from build123d import *

# Parameters (mm, degrees)
SKETCH_1_W          = 50
SKETCH_1_H          = 27
EXTRUDE_1_DEPTH     = 35
SKETCH_2_W          = 50
SKETCH_2_H          = 21
CUT_EXTRUDE_1_DEPTH = 15
SKETCH_3_R          = 1.6
CUT_EXTRUDE_2_DEPTH = 53.758784453
SKETCH_4_W          = 14
SKETCH_4_H          = 21
CUT_EXTRUDE_3_DEPTH = 63.544986529


with BuildPart() as part:
    # 草图1 → 凸台-拉伸1 (new body)
    with BuildSketch(Plane.XY):
        with Locations((3.800856531, -0.170235546)):
            Rectangle(SKETCH_1_W, SKETCH_1_H)
    extrude(amount=EXTRUDE_1_DEPTH)

    # 草图2 → 切除-拉伸1 (cut)
    with BuildSketch(Plane.XY.offset(35)):
        with Locations((3.800856531, -0.170235546)):
            Rectangle(SKETCH_2_W, SKETCH_2_H)
    extrude(amount=-CUT_EXTRUDE_1_DEPTH, mode=Mode.SUBTRACT)

    # 草图3 → 切除-拉伸2 (cut, through all)
    with BuildSketch(Plane.XZ.offset(13.670235546)):
        with Locations(Location((-3.699143469, 30, 0), (0, 0, 270))):
            Circle(SKETCH_3_R)
        with Locations(Location((11.300856531, 30, 0), (0, 0, 270))):
            Circle(SKETCH_3_R)
    extrude(amount=-CUT_EXTRUDE_2_DEPTH, mode=Mode.SUBTRACT)

    # 草图4 → 切除-拉伸3 (cut, through all)
    with BuildSketch(Plane.ZY.offset(21.199143469)):
        with Locations((10, -0.170235546)):
            Rectangle(SKETCH_4_W, SKETCH_4_H)
    extrude(amount=-CUT_EXTRUDE_3_DEPTH, mode=Mode.SUBTRACT)


solid = part.part
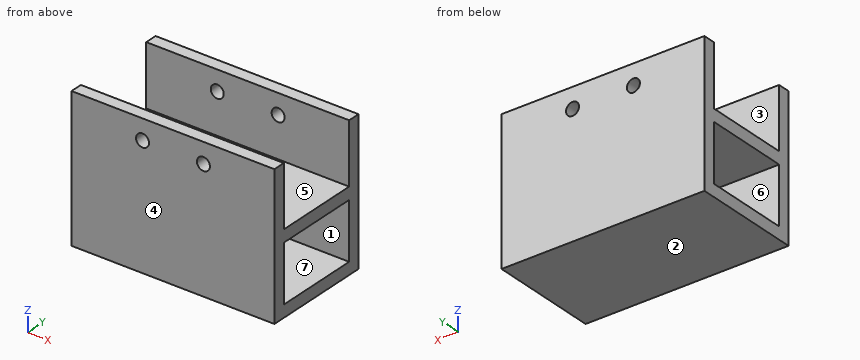
Check sheet for the modelled part. Datum: model origin and axes. Units: mm. Face numbers are marked on the shaded views. A direction names the side the tool comes from. Give positions to 0.01 mm unless a question says otherwise; leave off trailing zeros. Loops run counter-clockwise (first coordinate to the right, second up) from the corner with the lowest first, then second, coordinate; pieces in that order, holes last. Notation, with made-up numbers: M 9,10.25 L 36,10.25 A18 cw 36,43.25 Z; hole C 89.25,6.25 d2. An arc over 180 degrees is marked long. Return JSON: item names as keys, results as strings. Group by question number.
1. Thickness scan on L1, parallel to X at y = -11.5, z = 30; L2, parallel to Y at x = 2, z = 24; L3, parallel to Z at x = 18.5, y = -3. Record the ranges inside material, lowest first.
2. Cross-section at C-C on z = 30. Record the boundary of the cut face in (x, y), plus the area to 3 significant figures.
3. Mould release check, pull along Z, two halves, no side actions. Record for the marked faces 4, 5, 6 and 7: released by +Z, released by -Z, zero draft, split by the parting line, or undercut.
4. Cross-section at D-D on z = 15. Record the boundary of the cut face in (x, y).
5. Go/stop test with a flat-tipped pin: pin 1 (3 mm diameter, centred on x = -13.5, y = 8.5, fed in from +Z). Record where the tip stops, or that it passes through.
6. Cross-section at A-A on y = 5.25. Record the boundary of the cut face in (x, z).
7. Cross-section at B-B on x = 14. Record the boundary of the cut face in (y, z).
8. Tool access check on the marked faces 1, 2 and 3. Record the directions out of +Z, -Z, +X, -X, +Y, -Y that give a thin tool (end or side, any length) a straight path to the whole face; none if there is none.
Return value:
{
 "1": {"L1": "-21.2 to -5.3, -2.1 to 9.7, 12.9 to 28.8", "L2": "-13.67 to -10.67, 10.33 to 13.33", "L3": "0 to 3, 17 to 20"},
 "2": {"outline": "M -21.2,-13.67 L -5.3,-13.67 L -5.3,-10.67 L -21.2,-10.67 Z; M -21.2,10.33 L -5.3,10.33 L -5.3,13.33 L -21.2,13.33 Z; M -2.1,-13.67 L 9.7,-13.67 L 9.7,-10.67 L -2.1,-10.67 Z; M -2.1,10.33 L 9.7,10.33 L 9.7,13.33 L -2.1,13.33 Z; M 12.9,-13.67 L 28.8,-13.67 L 28.8,-10.67 L 12.9,-10.67 Z; M 12.9,10.33 L 28.8,10.33 L 28.8,13.33 L 12.9,13.33 Z", "area": "262 mm^2"},
 "3": {"face 4": "zero draft", "face 5": "released by +Z", "face 6": "undercut", "face 7": "undercut"},
 "4": {"outline": "M -21.2,-13.67 L 28.8,-13.67 L 28.8,-10.67 L -21.2,-10.67 Z; M -21.2,10.33 L 28.8,10.33 L 28.8,13.33 L -21.2,13.33 Z"},
 "5": {"pin 1": "z = 20"},
 "6": {"outline": "M -21.2,0 L 28.8,0 L 28.8,3 L -21.2,3 Z; M -21.2,17 L 28.8,17 L 28.8,20 L -21.2,20 Z"},
 "7": {"outline": "M -13.67,0 L 13.33,0 L 13.33,35 L 10.33,35 L 10.33,20 L -10.67,20 L -10.67,35 L -13.67,35 Z; hole M -10.67,3 L 10.33,3 L 10.33,17 L -10.67,17 Z"},
 "8": {"face 1": "+X, -X", "face 2": "-Z, +X, -X, +Y, -Y", "face 3": "+Z, +X, -X"}
}
